Input: dimensioned drawing with shaded views. Units: mm. Origin: part minimum x, y, z. Give positions to 0.01 mm unless a question says otherwise; leave off trailing zeros. Write each loop counter-clockwise with the first axis right and the second up, starting at its lowest first coordinate (ties: lowest second). Pieces come first, ordered by that corner, then holes. Notation, with made-up numbers: (-20, 64.5) - (38, 64.5) arc R18 ccw to (38, 73.5) - close; hole circle Ø3 at (-25, 2). An arc over 180 degrees is marked (long way). Answer as a JSON object with one key per item and string values. Group by question number.
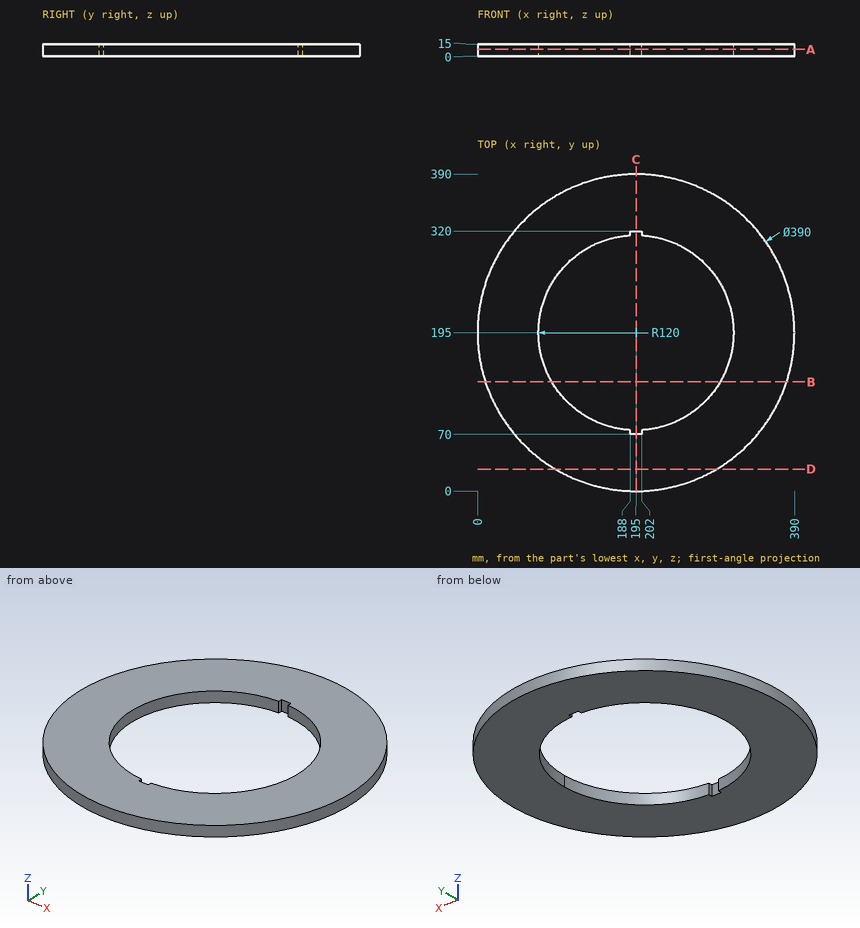
Q1. Section C-C on x = 195. Return the cut outline in (y, z).
Q2. First-contact query: pin 1 Ø5.5 at (y, z) = (73.5, 11) entering from +X; pin 2 Ø4 at (y, z) = (316.5, 4.5) entering from +X; pin 3 Ø1.6 at (y, z) = (73.5, 8) entering from -X. Flat tips, straight axial feed; report the tip coordinate or a pass-through.
Q3. Ray query, probe 1 along Y at (x, z) = (150, 10.5); probe 2 along Y at (x, z) = (199.5, 14.25); probe 3 along X at (y, z) = (120, 5). Return the intervals inside material, ascending. Write a range as [from, to].
Q4. Section A-A on z = 8.5. Return the cut outline in (x, y).
Q5. Section B-B on y = 134.5. Return the cut outline in (x, z).
Q6. Section D-D on y = 27. Return the cut outline in (x, z).
Taken from the geometry:
{
 "1": {"outline": "(0, 0) - (70, 0) - (70, 15) - (0, 15) - close; (320, 0) - (390, 0) - (390, 15) - (320, 15) - close"},
 "2": {"pin 1": "stops at x = 349.67", "pin 2": "stops at x = 349.09", "pin 3": "stops at x = 41.84"},
 "3": {"probe 1": "y = [5.26, 83.76], [306.24, 384.74]", "probe 2": "y = [0.05, 70], [320, 389.95]", "probe 3": "x = [15, 101.33], [288.67, 375]"},
 "4": {"outline": "circle Ø390 at (195, 195); hole (188, 70) - (202, 70) - (202, 75.2) arc R120 ccw to (315, 195) arc R120 ccw to (202, 314.8) - (202, 320) - (188, 320) - (188, 314.8) arc R120 ccw to (188, 75.2) - close"},
 "5": {"outline": "(9.62, 0) - (91.37, 0) - (91.37, 15) - (9.62, 15) - close; (298.63, 0) - (380.38, 0) - (380.38, 15) - (298.63, 15) - close"},
 "6": {"outline": "(96, 0) - (294, 0) - (294, 15) - (96, 15) - close"}
}
